The listing builds one solid part. Answer for the finished solid, in the listing's coordinates (mm). A direction names the side the tool comes from. Give positions to 0.01 mm unless a question says otherwise; leave off trailing zeros. Order: outer loops, then holes, each group sorted by start corner. A loop starts at its lowest first (then second) coordinate and runs counter-clockwise, first axis right, second up. Notation, with made-up numbers: (63, 68) - (80, 68) arc R16 ccw to (80, 87) - close; hole circle Ø11 at (-28.5, -9). An arc over 180 degrees is marked (long way). Answer as CSV lines item,"result". Start each with the question number.
1. Section D-D on y = 53 is taken. Give the vertices of the cut face in (x, z), and give its area (3 significant figures).
2. Determine the mould class of faces 1 (the cylindrical face through (67.43, -12.04, 2.71)), 2 (the flat face through (-5, 18, 7)), 3 (the flat face through (99, 17, 7)) for opening direction X: +X half, -X half, draft (parallel to the pull), parting line (faces both ways), or undercut.
3. Consider line 1 along Y through (x, z) = (94, 10.25); line 2 along X through (y, z) = (21, 4); line 3 along Z through (x, y) = (42, 5.5). Determine where each line is inside the solid, lowest interval first. Write a range as [from, to].
4. Which of the six approach directions +Z, -Z, +X, -X, +Y, -Y give full straight-line access (tool end or side, diameter ignored) to faces 4 (the flat face through (49, 10, 7.5)), 5 (the flat face through (55, 12, 5.5)), 6 (the cylindrical face through (0.703, 63.986, 7.148))?
5. Section A-A on z = 3 is taken. Give the vertices of the cut face in (x, y).
6. Flat-ended cylindrical pins translate along their axes: pin 1 (2 mm diameter, centred on x = 15, y = 18.5, fed in from -Z); pin 2 (17.5 mm diameter, centred on x = 47, y = 20, fed in from +Z); pin 3 (8 mm diameter, centred on x = 7, z = 12, fed in from +Y); pin 4 (8 mm diameter, centred on y = 60.5, z = 2, fed in from +X). Find the tip coordinate at first contact, or state that the pin passes through.
7. Section B-B on y = 20 is taken. Give the vertices of the cut face in (x, z).
8. Section C-C on x = 47 is taken. Give the vertices of the cut face in (y, z).
Autodesk Inventor part; units mm, degrees
ref_plane "YZ Plane" through (0, 0, 0) normal (1, 0, 0) x (0, 1, 0)
ref_plane "XZ Plane" through (0, 0, 0) normal (0, 1, 0) x (-1, 0, 0)
ref_plane "XY Plane" through (0, 0, 0) normal (0, 0, 1) x (1, 0, 0)
ref_plane "Work Plane1" through (0, 0, 0) normal (0, 0, 1) x (1, 0, 0)
sketch "Sketch1" plane through (0, 0, 0) normal (0, 0, 1) x (1, 0, 0)
  circle A0 centre (0, -5) radius 2
  circle A1 centre (94, 45) radius 2
  circle A2 centre (94, -5) radius 2
  circle A3 centre (0, 45) radius 2
  line L0 (5, -10) -> (5, 20)
  arc A4 (89, 20) -> (5, 20) centre (47, 20) ccw
  line L1 (89, 20) -> (89, -10)
  line L2 (99, -15) -> (99, 50)
  line L3 (79, 70) -> (15, 70)
  line L4 (-5, 50) -> (-5, -15)
  circle A5 centre (47, 20) radius 38
  circle A6 centre (77, 62) radius 4
  circle A7 centre (17, 62) radius 4
  line L5 (89, -10) -> (81, -10)
  line L6 (81, -20) -> (81, -10)
  line L7 (81, -20) -> (94, -20)
  line L8 (0, -20) -> (13, -20)
  line L9 (13, -20) -> (13, -10)
  line L10 (5, -10) -> (13, -10)
  line L11 (13, -20) -> (81, -20)
  arc A8 (94, -20) -> (99, -15) centre (94, -15) ccw
  arc A9 (99, 50) -> (79, 70) centre (79, 50) ccw
  arc A10 (15, 70) -> (-5, 50) centre (15, 50) ccw
  arc A11 (-5, -15) -> (0, -20) centre (0, -15) ccw
  point P0 (0, 0)
  dimension "d0" = 76
extrude "Extrusion1" add sketch "Sketch1" along normal blind 5.5 contours L10 L9 L8 A11 L4 A10 L3 A9 L2 A8 L7 L6 L5 L1 A4 L0 | L0 A4 L1 L5 L6 L11 L9 L10 | A6 | A7
sketch "Sketch2" plane through (0, 0, 5.5) normal (0, 0, 1) x (1, 0, 0)
  circle A0 centre (47, 20) radius 38
  circle A1 centre (0, 45) radius 2
  circle A2 centre (94, -5) radius 2
  circle A3 centre (94, 45) radius 2
  circle A4 centre (0, -5) radius 2
  line L0 (99, -15) -> (99, 50)
  line L1 (79, 70) -> (15, 70)
  line L2 (-5, 50) -> (-5, -15)
  circle A5 centre (47, 20) radius 10
  line L3 (0, -20) -> (94, -20)
  arc A6 (94, -20) -> (99, -15) centre (94, -15) ccw
  arc A7 (99, 50) -> (79, 70) centre (79, 50) ccw
  arc A8 (15, 70) -> (-5, 50) centre (15, 50) ccw
  arc A9 (-5, -15) -> (0, -20) centre (0, -15) ccw
  point P0 (0, 0)
  dimension "d3" = 20
extrude "Extrusion2" add sketch "Sketch2" along normal blind 2 contours A0 | A6 L3 A9 L2 A8 L1 A7 L0
sketch "Sketch3" plane through (0, 0, 7.5) normal (0, 0, 1) x (1, 0, 0)
  circle A0 centre (47, 20) radius 10
  circle A1 centre (0, -5) radius 2
  circle A2 centre (94, 45) radius 2
  circle A3 centre (94, -5) radius 2
  circle A4 centre (0, 45) radius 2
  line L0 (99, -15) -> (99, 50)
  line L1 (79, 70) -> (15, 70)
  line L2 (-5, 50) -> (-5, -15)
  circle A5 centre (47, 20) radius 11
  line L3 (0, -20) -> (94, -20)
  arc A6 (94, -20) -> (99, -15) centre (94, -15) ccw
  arc A7 (99, 50) -> (79, 70) centre (79, 50) ccw
  arc A8 (15, 70) -> (-5, 50) centre (15, 50) ccw
  arc A9 (-5, -15) -> (0, -20) centre (0, -15) ccw
  point P0 (0, 0)
  dimension "d6" = 22
extrude "Extrusion3" add sketch "Sketch3" along normal blind 7 contours A6 L3 A9 L2 A8 L1 A7 L0
sketch "Sketch4" plane through (0, 0, 0) normal (0, 0, -1) x (-1, 0, 0)
  circle A0 centre (0, -5) radius 2 construction
  circle A1 centre (-94, 45) radius 2 construction
  circle A2 centre (-94, -5) radius 2 construction
  circle A3 centre (0, 45) radius 2 construction
  line L0 (-85, -10) -> (-85, 20) construction
  arc A4 (-9, 20) -> (-85, 20) centre (-47, 20) ccw construction
  line L1 (-9, 20) -> (-9, -10) construction
  line L2 (5, -15) -> (5, 50) construction
  line L3 (-15, 70) -> (-79, 70) construction
  line L4 (-99, 50) -> (-99, -15) construction
  line L5 (-77, 62) -> (-17, 62) construction
  circle A5 centre (-77, 62) radius 4
  circle A6 centre (-17, 62) radius 4
  circle A7 centre (-77, 62) radius 4
  circle A8 centre (-17, 62) radius 4
  line L6 (-94, -20) -> (-81, -20)
  line L7 (-81, -20) -> (-81, -10)
  line L8 (-81, -10) -> (-85, -10)
  line L9 (-13, -10) -> (-9, -10)
  line L10 (-13, -20) -> (-13, -10)
  line L11 (0, -20) -> (-13, -20)
  arc A9 (-99, -15) -> (-94, -20) centre (-94, -15) ccw
  arc A10 (0, -20) -> (5, -15) centre (0, -15) ccw
  arc A11 (5, 50) -> (-15, 70) centre (-15, 50) ccw
  arc A12 (-79, 70) -> (-99, 50) centre (-79, 50) ccw
  point P0 (0, 0)
  point P1 (-47, 62)
  dimension "d9" = 8
  dimension "d10" = 8
  dimension "d11" = 60
extrude "Extrusion4" cut sketch "Sketch4" against normal through all
properties part number "frame bottom"
Checks:
1,outline,"(-4.77, 0) - (28.16, 0) - (28.16, 5.5) - (65.84, 5.5) - (65.84, 0) - (98.77, 0) - (98.77, 14.5) - (-4.77, 14.5) - close"
1,area,"1,290 mm²"
2,face 1,"undercut"
2,face 2,"-X half"
2,face 3,"+X half"
3,line 1,"y = [-20, -7], [-3, 43], [47, 63.23]"
3,line 2,"x = [-5, 9.01], [84.99, 99]"
3,line 3,"z = [5.5, 14.5]"
4,face 4,"+Z"
4,face 5,"-Z"
4,face 6,"+Z, -Z, -X, +Y"
5,outline,"(-5, -15) arc R5 ccw to (0, -20) - (94, -20) arc R5 ccw to (99, -15) - (99, 50) arc R20 ccw to (79, 70) - (15, 70) arc R20 ccw to (-5, 50) - close; hole circle Ø4 at (0, -5); hole circle Ø4 at (0, 45); hole circle Ø76 at (47, 20); hole circle Ø8 at (17, 62); hole circle Ø8 at (77, 62); hole circle Ø4 at (94, -5); hole circle Ø4 at (94, 45)"
6,pin 1,"stops at z = 5.5"
6,pin 2,"passes through"
6,pin 3,"stops at y = 69.6"
6,pin 4,"stops at x = 97.91"
7,outline,"(-5, 0) - (9, 0) - (9, 5.5) - (37, 5.5) - (37, 7.5) - (36, 7.5) - (36, 14.5) - (-5, 14.5) - close; (57, 5.5) - (85, 5.5) - (85, 0) - (99, 0) - (99, 14.5) - (58, 14.5) - (58, 7.5) - (57, 7.5) - close"
8,outline,"(-20, 0) - (-18, 0) - (-18, 5.5) - (10, 5.5) - (10, 7.5) - (9, 7.5) - (9, 14.5) - (-20, 14.5) - close; (30, 5.5) - (58, 5.5) - (58, 0) - (70, 0) - (70, 14.5) - (31, 14.5) - (31, 7.5) - (30, 7.5) - close"
